For this review, take the finished solid that the model builds, in its own axes (mm). Give positions to 0.01 mm unless a question says otherwise; leave off trailing zeros. Write each loop counter-clockwise with the first axis right and the second up, starting at its lowest first coordinate (ties: lowest second). Pieces come first, ordered by that corner, then holes. Notation, with made-up numbers: (44, 2) -> (73, 2) arc R25 ccw to (73, 26) -> close; hole circle Ø11 at (68.5, -23.75). An arc over 180 degrees is marked (long way). Return JSON: item names as keys, results as strings.
from build123d import *

# Parameters (mm, degrees)
BOSS_EXTRUDE1_DEPTH = 6.35
CUT_EXTRUDE1_REACH  = 8.35
SKETCH2_W           = 29.21
SKETCH2_H           = 29.21
FILLET1_R           = 5.08
BOSS_EXTRUDE2_DEPTH = 6.35
FILLET2_R           = 5.08


with BuildPart() as part:
    # Sketch1 → Boss-Extrude1 (new body)
    with BuildSketch(Plane.XY):
        with BuildLine():
            ThreePointArc((-79.739479369, 107.95), (-102.265174294, 55.997788823), (-107.940757138, -0.342489287))
            ThreePointArc((-107.940757138, -0.342489287), (0, -102.610284874), (107.940757138, -0.342489287))
            ThreePointArc((107.940757138, -0.342489287), (102.265174294, 55.997788823), (79.739479369, 107.95))
            ThreePointArc((79.739479369, 107.95), (0, 151.891393684), (-79.739479369, 107.95))
        make_face()
        with BuildLine():
            Line((-76.2, 101.6), (76.2, 101.6))
            ThreePointArc((76.2, 101.6), (96.55013665, 52.712534163), (101.6, 0))
            ThreePointArc((101.6, 0), (0, -96.260283012), (-101.6, 0))
            ThreePointArc((-101.6, 0), (-96.55013665, 52.712534163), (-76.2, 101.6))
        make_face(mode=Mode.SUBTRACT)
    extrude(amount=BOSS_EXTRUDE1_DEPTH)

    # Sketch2 → Cut-Extrude1 (cut, up to next)
    with BuildSketch(Plane.XY.offset(6.35), mode=Mode.PRIVATE) as cut_extrude1_sk1:
        with Locations((0, 126.745696842)):
            Rectangle(SKETCH2_W, SKETCH2_H)
    cut_extrude1_tool1 = extrude(cut_extrude1_sk1.sketch, amount=-CUT_EXTRUDE1_REACH, mode=Mode.PRIVATE) & part.part
    add(cut_extrude1_tool1.solids().sort_by_distance((0, 126.745697, 6.35))[0], mode=Mode.SUBTRACT)

    # Fillet1
    fillet1_edges = [part.edges().sort_by_distance(p)[0] for p in [
        (14.605, 141.350696842, 3.175),
        (14.605, 112.140696842, 3.175),
        (-14.605, 112.140696842, 3.175),
        (-14.605, 141.350696842, 3.175),
    ]]
    fillet(fillet1_edges, radius=FILLET1_R)

    # Sketch3 → Boss-Extrude2 (add)
    with BuildSketch(Plane.XY.offset(6.35)):
        Polygon((-77.659314664, 100.375489604), (69.28193291, -74.742270093), (72.200562238, -72.293249301), (-74.740685336, 102.824510396), align=None)
        Polygon((74.740685336, 102.824510396), (-72.200562238, -72.293249301), (-69.28193291, -74.742270093), (77.659314664, 100.375489604), align=None)
    extrude(amount=-BOSS_EXTRUDE2_DEPTH)

    # Fillet2
    fillet2_edges = [part.edges().sort_by_distance(p)[0] for p in [
        (73.713199114, 101.6, 3.175),
        (0, 13.752030134, 3.175),
        (-73.713199114, 101.6, 3.175),
        (-77.233836777, 99.868424803, 3.175),
        (-2.486800886, 10.788376244, 3.175),
        (-69.382552816, -68.934876448, 3.175),
        (-66.545991735, -71.481702369, 3.175),
        (0, 7.824722354, 3.175),
        (66.545991735, -71.481702369, 3.175),
        (69.382552816, -68.934876448, 3.175),
        (2.486800886, 10.788376244, 3.175),
        (77.233836777, 99.868424803, 3.175),
    ]]
    fillet(fillet2_edges, radius=FILLET2_R)


solid = part.part
1. For pin 1 (3 mm diameter, centred on y = -54, z = 0.5, fed in from +X); pin 2 (1.9 mm diameter, centred on x = 4, z = 4, fed in from -Y); pin 3 (3 mm diameter, centred on y = 123, z = 2, fed in from -X); pin 4 (1 mm diameter, centred on x = 77.5, y = 98, fed in from -Z), all flat-tipped, find the tip position at first contact; note any pin that passes through.
Results found:
{"pin 1": "stops at x = 91.23", "pin 2": "stops at y = -102.57", "pin 3": "stops at x = -69.35", "pin 4": "stops at z = 0"}
2. To check wall thickness, follow probe 1 along Y at (x, z) = (12, 4.25); probe 2 along X at (y, z) = (-62, 2); probe 3 along X at (y, z) = (-59.5, 2.5). State the ranges of each line that lie inside material, in increasing order.
Results found:
{"probe 1": "y = -101.94 to -95.55, -6.48 to -0.55, 22.13 to 28.05, 101.6 to 112.78, 140.71 to 151.12", "probe 2": "x = -84.44 to -76.15, -63.56 to -58.59, 58.59 to 63.56, 76.15 to 84.44", "probe 3": "x = -86.38 to -78.29, -61.47 to -56.49, 56.49 to 61.47, 78.29 to 86.38"}
3. Add section B-B, the plane y = 86. State the section outline as (x, z) points, plus the area to 3 significant figures.
Results found:
{"outline": "(-91.61, 0) -> (-84.6, 0) -> (-84.6, 6.35) -> (-91.61, 6.35) -> close; (-65.6, 0) -> (-60.62, 0) -> (-60.62, 6.35) -> (-65.6, 6.35) -> close; (60.62, 0) -> (65.6, 0) -> (65.6, 6.35) -> (60.62, 6.35) -> close; (84.6, 0) -> (91.61, 0) -> (91.61, 6.35) -> (84.6, 6.35) -> close", "area": "152 mm²"}
4. The part is to be moulded in two halves that separate along Y. For faces 1 (the cylindrical face through (-2.295, -102.586, 3.131)), 2 (the flat face through (-1, 16, 0)), 3 (the cylindrical face through (0.942, -96.256, 3.131)), say which applies: +Y half, -Y half, draft (parallel to the pull), parting line (faces both ways), or undercut.
Results found:
{"face 1": "-Y half", "face 2": "draft", "face 3": "undercut"}
5. Add section A-A, the plane x = 0. State the section outline as (y, z) points, plus the area to 3 significant figures.
Results found:
{"outline": "(-102.61, 0) -> (-96.26, 0) -> (-96.26, 6.35) -> (-102.61, 6.35) -> close; (5, 0) -> (16.58, 0) -> (16.58, 6.35) -> (5, 6.35) -> close; (101.6, 0) -> (112.14, 0) -> (112.14, 6.35) -> (101.6, 6.35) -> close; (141.35, 0) -> (151.89, 0) -> (151.89, 6.35) -> (141.35, 6.35) -> close", "area": "248 mm²"}
6. Add section D-D, the plane z = 4.75. Count the separate pieces of the cut face and the enclosed holes in it, plus the area to 3 significant figures.
Results found:
{"separate pieces": "1", "enclosed holes": "5", "area": "10,300 mm²"}
7. Add section C-C, the plane x = -86. State the section outline as (y, z) points, plus the area to 3 significant figures.
Results found:
{"outline": "(-60, 0) -> (-48.89, 0) -> (-48.89, 6.35) -> (-60, 6.35) -> close; (82.99, 0) -> (97.26, 0) -> (97.26, 6.35) -> (82.99, 6.35) -> close", "area": "161 mm²"}
